```python
from build123d import *

# Parameters (mm, degrees)
SKETCH1_W               = 64.389
SKETCH1_H               = 16.891
EXTRUDE1_DEPTH          = 57.4548
FILLET2_R               = 7.62
SHELL1_START            = 1.27
SHELL1_DEPTH            = 54.9148
CUT_EXTRUDE1_DEPTH      = 100.578641885
CUT_EXTRUDE1_DEPTH_BACK = 100.578641885
SKETCH4_W               = 0.889
SKETCH4_H               = 54.9148
EXTRUDE2_DEPTH          = 12.7
CUT_EXTRUDE2_DEPTH      = 20.32
CUT_EXTRUDE2_DEPTH_BACK = 19.05


# Read off the part's stored shape, not the designer's step: Shell1
with BuildPart() as part:
    # Sketch1 → Extrude1 (new body)
    with BuildSketch(Plane.XY):
        with Locations((-41.310464395, 26.366453204)):
            Rectangle(SKETCH1_W, SKETCH1_H)
    extrude(amount=EXTRUDE1_DEPTH)

    # Fillet2
    fillet2_edges = [part.edges().sort_by_distance(p)[0] for p in [
        (-73.504964395, 34.811953204, 28.7274),
        (-9.115964395, 34.811953204, 28.7274),
    ]]
    fillet(fillet2_edges, radius=FILLET2_R)

    # Shell1 outline → Shell1 (cut)
    with BuildSketch(Plane.XY.offset(SHELL1_START)):
        with BuildLine():
            Line((-16.735964395, 33.541953204), (-16.735964395, 34.811953204))
            Line((-16.735964395, 34.811953204), (-65.884964395, 34.811953204))
            Line((-65.884964395, 34.811953204), (-65.884964395, 33.541953204))
            ThreePointArc((-65.884964395, 33.541953204), (-70.375092455, 31.682081264), (-72.234964395, 27.191953204))
            Line((-72.234964395, 27.191953204), (-72.234964395, 19.190953204))
            Line((-72.234964395, 19.190953204), (-10.385964395, 19.190953204))
            Line((-10.385964395, 19.190953204), (-10.385964395, 27.191953204))
            ThreePointArc((-10.385964395, 27.191953204), (-12.245836334, 31.682081265), (-16.735964395, 33.541953204))
        make_face()
    extrude(amount=SHELL1_DEPTH, mode=Mode.SUBTRACT)

    # Sketch2 → Cut-Extrude1 (cut, two sides: drawn at the far end of the back side and taken through both)
    with BuildSketch(Plane(origin=(0, 0, 0), x_dir=(0, 0, -1), z_dir=(1, 0, 0)).offset(-CUT_EXTRUDE1_DEPTH_BACK)):
        with BuildLine():
            Line((-189.674707518, 34.811953204), (-58.293, 34.811953204))
            Line((-58.293, 34.811953204), (-55.698725793, 34.811953204))
            Line((-55.698725793, 34.811953204), (-55.698725793, 26.937953204))
            ThreePointArc((-55.698725793, 26.937953204), (-55.401146283, 26.219532715), (-54.682725793, 25.921953204))
            Line((-54.682725793, 25.921953204), (-54.428725793, 25.921953204))
            ThreePointArc((-54.428725793, 25.921953204), (-53.530700181, 26.293927592), (-53.158725793, 27.191953204))
            Line((-53.158725793, 27.191953204), (-53.158725793, 34.811953204))
            Line((-53.158725793, 34.811953204), (-36.648725793, 34.811953204))
            Line((-36.648725793, 34.811953204), (-36.648725793, 27.191953204))
            ThreePointArc((-36.648725793, 27.191953204), (-36.276751405, 26.293927592), (-35.378725793, 25.921953204))
            Line((-35.378725793, 25.921953204), (-21.916725793, 25.921953204))
            ThreePointArc((-21.916725793, 25.921953204), (-21.018700181, 26.293927592), (-20.646725793, 27.191953204))
            Line((-20.646725793, 27.191953204), (-20.646725793, 34.811953204))
            Line((-20.646725793, 34.811953204), (-4.136725793, 34.811953204))
            Line((-4.136725793, 34.811953204), (-4.136725793, 26.937953204))
            ThreePointArc((-4.136725793, 26.937953204), (-3.839146283, 26.219532715), (-3.120725793, 25.921953204))
            Line((-3.120725793, 25.921953204), (-2.612725793, 25.921953204))
            ThreePointArc((-2.612725793, 25.921953204), (-1.894305303, 26.219532715), (-1.596725793, 26.937953204))
            Line((-1.596725793, 26.937953204), (-1.596725793, 34.811953204))
            Line((-1.596725793, 34.811953204), (0, 34.811953204))
            Line((0, 34.811953204), (131.381707518, 34.811953204))
            Line((131.381707518, 34.811953204), (131.381707518, 297.575368241))
            Line((131.381707518, 297.575368241), (-189.674707518, 297.575368241))
            Line((-189.674707518, 297.575368241), (-189.674707518, 34.811953204))
        make_face()
    extrude(amount=CUT_EXTRUDE1_DEPTH + CUT_EXTRUDE1_DEPTH_BACK, mode=Mode.SUBTRACT)

    # Sketch4 → Extrude2 (add)
    with BuildSketch(Plane(origin=(0, 19.190953204, 0), x_dir=(-1, 0, 0), z_dir=(0, 1, 0))):
        with Locations((40.675464395, 28.7274)):
            Rectangle(SKETCH4_W, SKETCH4_H)
        with Locations((25.308464395, 28.7274)):
            Rectangle(SKETCH4_W, SKETCH4_H)
        with Locations((56.042464395, 28.7274)):
            Rectangle(SKETCH4_W, SKETCH4_H)
    extrude(amount=EXTRUDE2_DEPTH)

    # Sketch5 → Cut-Extrude2 (cut, two sides: drawn at the far end of the back side and taken through both)
    with BuildSketch(Plane.ZY.offset(41.119964395).offset(-CUT_EXTRUDE2_DEPTH_BACK)):
        Polygon((1.27, 31.890953204), (11.7729, 24.524953204), (45.6819, 24.524953204), (56.1848, 31.890953204), align=None)
    extrude(amount=CUT_EXTRUDE2_DEPTH + CUT_EXTRUDE2_DEPTH_BACK, mode=Mode.SUBTRACT)


solid = part.part
```
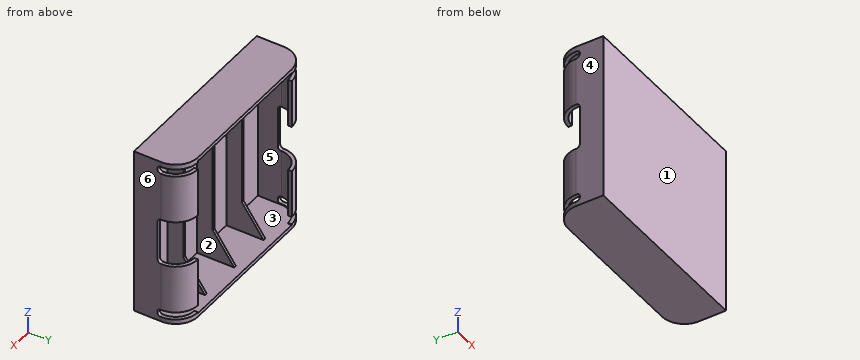
Work out the finished part from the listing and answer in its coordinate system (mm). Face numbers are marked on the shaded views. A direction names the side the tool comes from. Round coordinates to 2 decimals unless told otherwise and drop trailing zeros. Loops run counter-clockwise (first coordinate to the right, second up) from the corner with the lowest first, then second, coordinate; pieces in that order, holes last.
(1) The part is cut by section B-B, the plane y = 23. Give the vertices of the cut face in (x, z).
Computed values:
outline: (-73.5, 0) - (-9.12, 0) - (-9.12, 57.45) - (-73.5, 57.45) - close; hole (-72.23, 1.27) - (-56.49, 1.27) - (-56.49, 56.18) - (-72.23, 56.18) - close; hole (-55.6, 1.27) - (-41.12, 1.27) - (-41.12, 56.18) - (-55.6, 56.18) - close; hole (-40.23, 1.27) - (-25.75, 1.27) - (-25.75, 56.18) - (-40.23, 56.18) - close; hole (-24.86, 1.27) - (-10.39, 1.27) - (-10.39, 56.18) - (-24.86, 56.18) - close
(2) For the marked faces 1 and 2, determine the directions among +Z, -Z, +X, -X, +Y, -Y from which every point of the face is accessible in a straight line to the end or side of a thin tool.
Computed values:
face 1: +Z, -Z, +X, -X, -Y
face 2: +Y
(3) The part is cut by section D-D, the plane x = -52. Give the vertices of the cut face in (y, z), and give its area (3 significant figures).
Computed values:
outline: (17.92, 0) - (34.81, 0) - (34.81, 1.27) - (19.19, 1.27) - (19.19, 56.18) - (34.81, 56.18) - (34.81, 57.45) - (17.92, 57.45) - close
area: 113 mm2
(4) The part is cut by section C-C, the plane z = 41.5. Give the vertices of the cut face in (x, y), and give its area (3 significant figures).
Computed values:
outline: (-73.5, 17.92) - (-9.12, 17.92) - (-9.12, 27.19) arc R7.62 ccw to (-16.74, 34.81) - (-16.74, 33.54) arc R6.35 cw to (-10.39, 27.19) - (-10.39, 19.19) - (-24.86, 19.19) - (-24.86, 24.52) - (-25.75, 24.52) - (-25.75, 19.19) - (-40.23, 19.19) - (-40.23, 24.52) - (-41.12, 24.52) - (-41.12, 19.19) - (-55.6, 19.19) - (-55.6, 24.52) - (-56.49, 24.52) - (-56.49, 19.19) - (-72.23, 19.19) - (-72.23, 27.19) arc R6.35 cw to (-65.88, 33.54) - (-65.88, 34.81) arc R7.62 ccw to (-73.5, 27.19) - close
area: 144 mm2
(5) The mould has two halves that part along X. Classify the marked faces 3, 4, 5 and 6: pulls with the +X half, pulls with the -X half, needs draft (parallel to the pull), parting line crosses it, or undercut.
Computed values:
face 3: undercut
face 4: pulls with the -X half
face 5: undercut
face 6: pulls with the +X half
(6) The part is cut by section A-A, the plane x = -12.5. Give the vertices of the cut face in (y, z), and give its area (3 significant figures).
Computed values:
outline: (17.92, 0) - (33.53, 0) - (33.53, 1.6) - (31.92, 1.6) - (31.92, 1.27) - (19.19, 1.27) - (19.19, 56.18) - (31.92, 56.18) - (31.92, 55.7) - (33.53, 55.7) - (33.53, 57.45) - (17.92, 57.45) - close; (31.92, 4.14) - (33.53, 4.14) - (33.53, 20.65) - (31.92, 20.65) - close; (31.92, 36.65) - (33.53, 36.65) - (33.53, 53.16) - (31.92, 53.16) - close
area: 164 mm2
(7) Find the intervals of material crossed by L1, parallel to X at y = 25.5, z = 55; L2, parallel to Z at x = -55.5, y = 23.5; L3, parallel to X at y = 30.5, z = 45, in increasing order.
Computed values:
L1: x = -73.5 to -72.23, -56.49 to -55.6, -41.12 to -40.23, -25.75 to -24.86, -10.39 to -9.12
L2: z = 0 to 1.27, 56.18 to 57.45
L3: x = -72.75 to -71.31, -11.32 to -9.87
(8) Each of these flat-tipped pins is pushed along its axis until it touches: P1, Ø5, axis at y = 29.5, z = 26, coming from the -X side; P2, Ø0.5, axis at y = 34, z = 56, coming from the -X side; P3, Ø11.5, axis at x = -32, z = 33, coming from the +Y side. Where does it stop, or does it pass through?
Computed values:
P1: passes through
P2: stops at x = -69.77
P3: stops at y = 19.19
